CAD build for the part. Positions are in the model's coordinates, mm. A direction names the side the tool comes from. Give positions to 0.01 mm unless a question says otherwise; leave off trailing zeros. Write each loop counter-clockwise with the first axis right and the second up, starting at its lowest first coordinate (ties: lowest second). Pieces come first, ordered by that corner, then holes. Notation, with made-up numbers: (-11.5, 44.25) - (18.5, 44.25) arc R13 cw to (18.5, 67.25) - close; hole circle Ø3 at (-22, 53.5). An arc over 180 degrees is marked (long way). Answer as a JSON object with one key per item and string values.
from build123d import *

# Parameters (mm, degrees)
SKETCH1_R                = 4.5
BOSS_EXTRUDE1_DEPTH      = 10
BOSS_EXTRUDE2_DEPTH      = 22
BOSS_EXTRUDE2_DEPTH_BACK = 48
BOSS_EXTRUDE3_START      = -48
BOSS_EXTRUDE3_DEPTH      = 48
SKETCH5_R                = 8
CUT_EXTRUDE1_DEPTH       = 54


with BuildPart() as part:
    # Sketch1 → Boss-Extrude1 (new body)
    with BuildSketch(Plane.XY):
        with BuildLine():
            Line((-38, -14), (38, -14))
            ThreePointArc((38, -14), (50.215198798, -6.840242563), (49.936417534, 7.315868811))
            Line((49.936417534, 7.315868811), (11.936417534, 69.315868811))
            ThreePointArc((11.936417534, 69.315868811), (0, 76), (-11.936417534, 69.315868811))
            Line((-11.936417534, 69.315868811), (-49.936417534, 7.315868811))
            ThreePointArc((-49.936417534, 7.315868811), (-50.215198798, -6.840242563), (-38, -14))
        make_face()
        with Locations((0, 62)):
            Circle(SKETCH1_R, mode=Mode.SUBTRACT)
        with Locations((38, 0)):
            Circle(SKETCH1_R, mode=Mode.SUBTRACT)
        with Locations(Location((-38, 0, 0), (0, 0, 180))):
            Circle(SKETCH1_R, mode=Mode.SUBTRACT)
    extrude(amount=BOSS_EXTRUDE1_DEPTH)

    # Sketch2 → Boss-Extrude2 (add, two sides: drawn at the far end of the back side and taken through both)
    with BuildSketch(Plane.XZ.offset(14).offset(-BOSS_EXTRUDE2_DEPTH_BACK)):
        with BuildLine():
            ThreePointArc((-16.5, 24), (-14.427925282, 15.994691008), (-8.732124598, 10))
            Line((-8.732124598, 10), (8.732124598, 10))
            ThreePointArc((8.732124598, 10), (14.427925282, 15.994691008), (16.5, 24))
            ThreePointArc((16.5, 24), (0, 40.5), (-16.5, 24))
        make_face()
        with BuildLine():
            Line((8.732124598, 10), (-8.732124598, 10))
            ThreePointArc((-8.732124598, 10), (0, 7.5), (8.732124598, 10))
        make_face()
    extrude(amount=BOSS_EXTRUDE2_DEPTH + BOSS_EXTRUDE2_DEPTH_BACK)

    # Sketch2_3 → Boss-Extrude3 (add)
    with BuildSketch(Plane.XZ.offset(14).offset(BOSS_EXTRUDE3_START)):
        with BuildLine():
            ThreePointArc((16.5, 24), (14.427925282, 15.994691008), (8.732124598, 10))
            Line((8.732124598, 10), (16.5, 10))
            Line((16.5, 10), (16.5, 24))
        make_face()
        with BuildLine():
            Line((-16.5, 24), (-16.5, 10))
            Line((-16.5, 10), (-8.732124598, 10))
            ThreePointArc((-8.732124598, 10), (-14.427925282, 15.994691008), (-16.5, 24))
        make_face()
    extrude(amount=BOSS_EXTRUDE3_DEPTH)

    # Sketch5 → Cut-Extrude1 (cut)
    with BuildSketch(Plane.XZ.offset(36)):
        with Locations((0, 24)):
            Circle(SKETCH5_R)
    extrude(amount=-CUT_EXTRUDE1_DEPTH, mode=Mode.SUBTRACT)


solid = part.part
(1) 3-axis set-ups, long thin cutter, end or side, ignore diameter. For faces 5 (the face through (0, 34, 25)), 6 (the face through (-1.041, -9.378, 31.932)), 7 (the face through (-30.7, 38.7, 4.9)), 8 (the face through (42.292, 1.352, 4.93)), 9 (the face through (16.5, 10, 17)): which of +Z, -Z, +X, -X, +Y, -Y reach the whole face in a straight line?
Answer key:
{"face 5": "+Z, +X, -X, +Y", "face 6": "-Y", "face 7": "+Z, -Z, -X, +Y", "face 8": "+Z, -Z", "face 9": "+Z, +X, +Y, -Y"}
(2) Pull direction Y, two halves, no side cores. Call faces 1 (the face through (-16.5, 10, 17)), 2 (the face through (-1, -14, 7)), 3 (the face through (-50.315, -6.658, 4.93)), 4 (the face through (2.419, 65.794, 4.93)): pulls with the +Y half, pulls with the -Y half, needs draft (parallel to the pull), parting line crosses it, or undercut.
Answer key:
{"face 1": "needs draft", "face 2": "pulls with the -Y half", "face 3": "parting line crosses it", "face 4": "undercut"}
(3) Saw through at B-B, the plane x = 0. Give the cut face in (y, z).
Answer key:
{"outline": "(-36, 7.5) - (-14, 7.5) - (-14, 0) - (57.5, 0) - (57.5, 10) - (34, 10) - (34, 40.5) - (-36, 40.5) - (-36, 32) - (18, 32) - (18, 16) - (-36, 16) - close; (66.5, 0) - (76, 0) - (76, 10) - (66.5, 10) - close"}
(4) Saw through at C-C, the plane z = 5. Give the cut face in (x, y), and give its area (3 significant figures).
Answer key:
{"outline": "(-49.94, 7.32) arc R14 ccw to (-38, -14) - (38, -14) arc R14 ccw to (49.94, 7.32) - (11.94, 69.32) arc R14 ccw to (-11.94, 69.32) - close; hole circle Ø9 at (-38, 0); hole circle Ø9 at (0, 62); hole circle Ø9 at (38, 0)", "area": "5,880 mm²"}
(5) Saw through at D-D, the plane y = 62. Give the cut face in (x, z), and give its area (3 significant figures).
Answer key:
{"outline": "(-16.42, 0) - (-4.5, 0) - (-4.5, 10) - (-16.42, 10) - close; (4.5, 0) - (16.42, 0) - (16.42, 10) - (4.5, 10) - close", "area": "238 mm²"}
(6) Probe L1, parallel to X at y = -0.5, z = 3.5; L2, parallel to Z at x = 0, y = -20.5; L3, parallel to Y at x = 0, z = 6.5. List the from-to ranges inside material, lowest first. Write a range as [from, to].
Answer key:
{"L1": "x = [-51.99, -42.47], [-33.53, 33.53], [42.47, 51.99]", "L2": "z = [7.5, 16], [32, 40.5]", "L3": "y = [-14, 57.5], [66.5, 76]"}
(7) Flat gauge pins, fed straight in: P1, Ø4, axis at y = 3.5, z = 31, coming from the -X side; P2, Ø18.5, axis at x = 0, z = 24, coming from the +Y side; P3, Ø6, axis at y = 37.5, z = 22, coming from the -X side; P4, Ø7, axis at y = 1, z = 16.5, coming from the +X side. Where does each tip first touch, or does it go through?
Answer key:
{"P1": "stops at x = -15.72", "P2": "stops at y = 34", "P3": "passes through", "P4": "stops at x = 16.5"}
(8) Saw through at A-A, the plane y = 2.5. Give the cut face in (x, z).
Answer key:
{"outline": "(-51.77, 0) - (-41.74, 0) - (-41.74, 10) - (-51.77, 10) - close; (-34.26, 0) - (34.26, 0) - (34.26, 10) - (16.5, 10) - (16.5, 24) arc R16.5 ccw to (-16.5, 24) - (-16.5, 10) - (-34.26, 10) - close; (41.74, 0) - (51.77, 0) - (51.77, 10) - (41.74, 10) - close; hole circle Ø16 at (0, 24)"}
